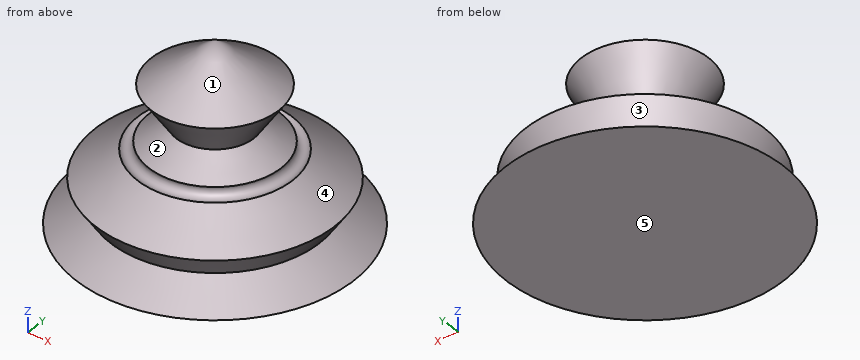
from build123d import *

# Parameters (mm, degrees)
F2_R = 2.5


with BuildPart() as f1:
    # F0 (on Front) → F1 (revolve)
    with BuildSketch(Plane.XZ):
        Polygon((0, 65.34344), (0, 0), (50.819985, 0), (38.281162, 8.357699), (43.692497, 16.476175), (14.215877, 36.123689), (23.327958, 49.79429), align=None)
    revolve(axis=Axis((0, 0, 32.67172), (0, 0, 1)))

    # F2 (on Right) → F3 (revolve, cut)
    with BuildSketch(Plane.YZ):
        with Locations((26.287429, 28.140074)):
            Circle(F2_R)
    revolve(axis=Axis((0, 0, 32.67172), (0, 0, 1)), mode=Mode.SUBTRACT)


solid = f1.part
Could you check a few things on this model? Use its own coordinates, in mm. Face numbers are marked on the shaded views. A direction names the side the tool comes from. Give positions to 0.01 mm unless a question says otherwise; leave off trailing zeros. Order: outer loops, then holes, each group sorted by start corner. A loop starts at its lowest first (then second) coordinate and runs counter-clockwise, first axis right, second up. Notation, with made-up numbers: (-7.75, 74.25) - (36.25, 74.25) arc R10 ccw to (36.25, 85.25) - close; hole circle Ø1 at (67, 73.25). An arc over 180 degrees is marked (long way). Return JSON: item names as keys, results as strings. Group by question number.
Q1. Which directions (+Z, -Z, +X, -X, +Y, -Y) give clear straight access to the entire face, cutting with the end or side of a thin tool? Please do the marked faces 1 and 2.
Q2. Will these pins go through, and if not, where does the flat tip stop? pin 1 Ø6 at (x, y) = (18.5, 31.5) entering from +Z; pin 2 Ø5 at (y, z) = (-16.5, 53.5) entering from +X; pin 3 Ø3 at (y, z) = (-14.5, 29) entering from +X.
Q3. Thinking about a two-plate mould opening in Z: for the marked faces 3, 4 and 5, which applies, pulls with the +Z half, pulls with the -Z half, needs draft (parallel to the pull), parting line crosses it, or undercut?
Q4. Please list where these lines run through material, in increasing order: line 1 along Z through (x, y) = (-26, 1); line 2 along Z through (x, y) = (-14, -15); line 3 along Z through (x, y) = (14, 38.5). Write a range as [from, to].
Q5. Suppose I cut it at B-B, the plane z = 7. Please give me the cut outline in (x, y).
Q6. Suppose I cut it at A-A, the plane z = 24. Please give me the cut outline in (x, y).
Resolved:
{
 "1": {"face 1": "+Z", "face 2": "none"},
 "2": {"pin 1": "stops at z = 23.25", "pin 2": "stops at x = 14.48", "pin 3": "stops at x = 20.34"},
 "3": {"face 3": "undercut", "face 4": "pulls with the +Z half", "face 5": "pulls with the -Z half"},
 "4": {"line 1": "z = [0, 25.65]", "line 2": "z = [0, 31.92], [45.58, 51.67]", "line 3": "z = [0, 6.57], [12.39, 18.29]"},
 "5": {"outline": "circle Ø80.64 at (0, 0)"},
 "6": {"outline": "circle Ø64.81 at (0, 0)"}
}
